from build123d import *

# Parameters (mm, degrees)
CYLINDER064_R     = 1
CYLINDER064_DEPTH = 20
CYLINDER065_R     = 1
CYLINDER065_DEPTH = 20
CYLINDER066_R     = 7
CYLINDER066_DEPTH = 1


with BuildPart() as obj1:
    # Cylinder064 → Cylinder064 (new body)
    with BuildSketch(Plane(origin=(-3.5, -3.5, 0), x_dir=(1, 0, 0), z_dir=(0, 0, 1))):
        Circle(CYLINDER064_R)
    extrude(amount=CYLINDER064_DEPTH)


with BuildPart() as compound035:
    # Cylinder065 → Cylinder065 (new body)
    with BuildSketch(Plane(origin=(3.5, 3.5, 0), x_dir=(1, 0, 0), z_dir=(0, 0, 1))):
        Circle(CYLINDER065_R)
    extrude(amount=CYLINDER065_DEPTH)

    # Compound035: union obj1
    add(obj1.part)


with BuildPart() as cut035:
    # Cylinder066 → Cylinder066 (new body)
    with BuildSketch(Plane.XY.offset(10)):
        Circle(CYLINDER066_R)
    extrude(amount=CYLINDER066_DEPTH)

    # Cut035: cut Compound035
    add(compound035.part, mode=Mode.SUBTRACT)


solid = cut035.part
Source: CAD feature listing. Evaluate the final solid. Frame: model axes, mm. Round coordinates to 2 decimals unless told otherwise and drop trailing zeros. Loops run counter-clockwise (first coordinate to the right, second up) from the corner with the lowest first, then second, coordinate; pieces in that order, holes last. Notation, with made-up numbers: M 17,4.25 L 56,4.25 A22 cw 56,16.25 Z; hole C 55.5,-34.5 d8. An arc over 180 degrees is marked long. Return JSON: item names as keys, results as strings. Group by question number.
1. Mould query, pull axis X, two halves, no side actions, for faces 1 (the face through (-4.5, -3.5, 10.5)), 2 (the face through (0, 0, 11)), 3 (the face through (6.466, -2.681, 10.493)). Classes: released by +X, released by -X, zero draft, split by the parting line, or undercut.
2. Section query B-B on z = 10.6. Output: boundary loops of the cut face in (x, y), and give its area (3 significant figures).
3. Section query C-C on y = -3.25. Output: boundary loops of the cut face in (x, z), and give its area (3 significant figures).
4. Material intervals for line 1 along X through (y, z) = (-3.5, 10.2); line 2 along X through (y, z) = (-3, 10.55); line 3 along Y through (x, z) = (3, 10.5), sorted ascending. Write a range as from..to.
5. Section query D-D on y = 1.5. Output: boundary loops of the cut face in (x, z), and give its area (3 significant figures).
6. Section query A-A on x = 3. Output: boundary loops of the cut face in (y, z), and give its area (3 significant figures).
Checks:
{
 "1": {"face 1": "undercut", "face 2": "zero draft", "face 3": "split by the parting line"},
 "2": {"outline": "C 0,0 d14; hole C -3.5,-3.5 d2; hole C 3.5,3.5 d2", "area": "148 mm²"},
 "3": {"outline": "M -6.2,10 L -4.47,10 L -4.47,11 L -6.2,11 Z; M -2.53,10 L 6.2,10 L 6.2,11 L -2.53,11 Z", "area": "10.5 mm²"},
 "4": {"line 1": "x = -6.06..-4.5, -2.5..6.06", "line 2": "x = -6.32..-4.37, -2.63..6.32", "line 3": "y = -6.32..2.63, 4.37..6.32"},
 "5": {"outline": "M -6.84,10 L 6.84,10 L 6.84,11 L -6.84,11 Z", "area": "13.7 mm²"},
 "6": {"outline": "M -6.32,10 L 2.63,10 L 2.63,11 L -6.32,11 Z; M 4.37,10 L 6.32,10 L 6.32,11 L 4.37,11 Z", "area": "10.9 mm²"}
}
